Source: three-view drawing plus pictorial views. Frame: mm from the lowest corner of the part. Give positions to 0.01 mm unless a question says otherwise; leave off trailing zeros. Order: outer loops, then holes, each group sorted by start corner. A loop starts at its lowest first (then second) coordinate and runs counter-clockwise, first axis right, second up. Notation, with made-up numbers: (-21, -19.5) -> (-3, -19.5) arc R5 cw to (-3, -15.5) -> close; hole circle Ø11 at (74.25, 76.5). An arc over 180 degrees is marked (long way). Use a Markdown table: item, result. Add a question column.
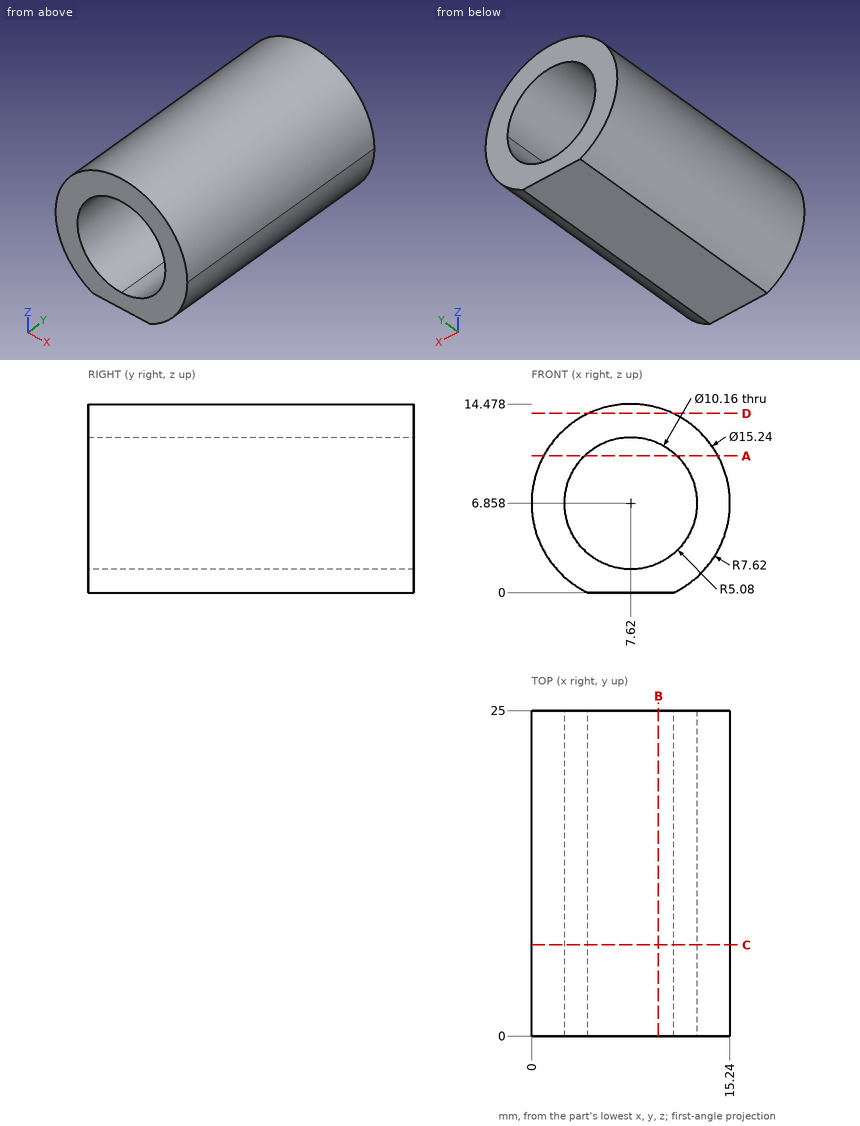
Q1. Section query D-D (z = 13.75). Return loops of the section in (x, y).
Q2. Section query C-C (y = 7). Return loops of the section in (x, z).
Q3. Section query A-A (z = 10.5). Return loops of the section in (x, y), plus the area to 3 significant figures.
Q4. First-contact query: pin 1 (2 mm diameter, centred on y = 4.5, z = 9, fed in from +X); pin 2 (2 mm diameter, centred on x = 1.5, y = 21.5, fed in from +Z); pin 3 (1.5 mm diameter, centred on y = 4, z = 4, fed in from -X). Flat tips, straight axial feed; report the tip coordinate or a pass-through.
Q5. Section query B-B (x = 9.75). Return loops of the section in (y, z).
Q6. Ray query, line 1 (X direction, y = 19.5, z = 10.75); line 2 (Z direction, x = 3.75, y = 17); line 3 (X direction, y = 6.5, z = 3.25). Return the intervals inside material, ascending.
Solution:
| question | item | result |
|---|---|---|
| 1 | outline | (4.37, 0) -> (10.87, 0) -> (10.87, 25) -> (4.37, 25) -> close |
| 2 | outline | (4.3, 0) -> (10.94, 0) arc R7.62 ccw to (15.24, 6.86) arc R7.62 ccw (long way) to start; hole (7.62, 1.78) arc R5.08 ccw to (12.7, 6.86) arc R5.08 ccw (long way) to start |
| 3 | outline | (0.93, 0) -> (4.08, 0) -> (4.08, 25) -> (0.93, 25) -> close; (11.16, 0) -> (14.31, 0) -> (14.31, 25) -> (11.16, 25) -> close |
| 3 | area | 158 mm² |
| 4 | pin 1 | stops at x = 15.15 |
| 4 | pin 2 | stops at z = 12.5 |
| 4 | pin 3 | stops at x = 0.3 |
| 5 | outline | (0, 0) -> (25, 0) -> (25, 2.25) -> (0, 2.25) -> close; (0, 11.47) -> (25, 11.47) -> (25, 14.17) -> (0, 14.17) -> close |
| 6 | line 1 | x = 1.07 to 4.36, 10.88 to 14.17 |
| 6 | line 2 | z = 0.29 to 3.57, 10.15 to 13.42 |
| 6 | line 3 | x = 0.91 to 4.04, 11.2 to 14.33 |
